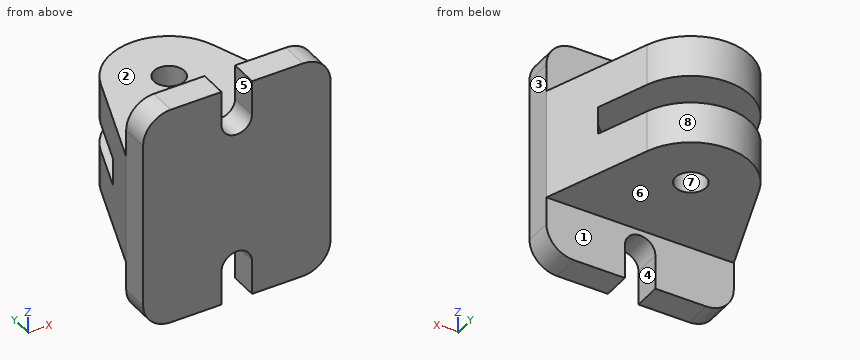
from build123d import *

# Parameters (mm, degrees)
SKETCH1_R           = 2.75
BOSS_EXTRUDE1_DEPTH = 10
SKETCH2_R           = 14.5
CUT_EXTRUDE1_DEPTH  = 2.5
BOSS_EXTRUDE2_DEPTH = 5
CUT_EXTRUDE5_DEPTH  = 41.387552571


with BuildPart() as part:
    # Sketch1 → Boss-Extrude1 (new, symmetric)
    with BuildSketch(Plane.XY):
        with BuildLine():
            Line((-10.101695673, 3.676716541), (-16.899464568, -15))
            Line((-16.899464568, -15), (16.899464568, -15))
            Line((16.899464568, -15), (10.101695673, 3.676716541))
            ThreePointArc((10.101695673, 3.676716541), (0, 10.75), (-10.101695673, 3.676716541))
        make_face()
        Circle(SKETCH1_R, mode=Mode.SUBTRACT)
    extrude(amount=BOSS_EXTRUDE1_DEPTH, both=True)

    # Sketch2 → Cut-Extrude1 (cut, symmetric)
    with BuildSketch(Plane.XY):
        Circle(SKETCH2_R)
    extrude(amount=CUT_EXTRUDE1_DEPTH, both=True, mode=Mode.SUBTRACT)

    # Sketch3 → Boss-Extrude2 (add)
    with BuildSketch(Plane.XZ.offset(15)):
        with BuildLine():
            Line((-16.899464568, 15), (-16.899464568, 10))
            Line((-16.899464568, 10), (16.899464568, 10))
            Line((16.899464568, 10), (16.899464568, 15))
            ThreePointArc((16.899464568, 15), (15.434998474, 18.535533906), (11.899464568, 20))
            Line((11.899464568, 20), (-11.899464568, 20))
            ThreePointArc((-11.899464568, 20), (-15.434998474, 18.535533906), (-16.899464568, 15))
        make_face()
        Polygon((16.899464568, 10), (-16.899464568, 10), (-16.899464568, -10), (16.899464568, -10), (16.899464568, 0), align=None)
        with BuildLine():
            Line((16.899464568, -10), (-16.899464568, -10))
            Line((-16.899464568, -10), (-16.899464568, -15))
            ThreePointArc((-16.899464568, -15), (-15.434998474, -18.535533906), (-11.899464568, -20))
            Line((-11.899464568, -20), (11.899464568, -20))
            ThreePointArc((11.899464568, -20), (15.434998474, -18.535533906), (16.899464568, -15))
            Line((16.899464568, -15), (16.899464568, -10))
        make_face()
    extrude(amount=BOSS_EXTRUDE2_DEPTH)

    # Sketch4 → Cut-Extrude5 (cut, through all)
    with BuildSketch(Plane.XZ.offset(20)):
        with BuildLine():
            Line((-2.75, 20), (-2.75, 13.75))
            ThreePointArc((-2.75, 13.75), (0, 11), (2.75, 13.75))
            Line((2.75, 13.75), (2.75, 20))
            Line((2.75, 20), (-2.75, 20))
        make_face()
        with BuildLine():
            Line((-2.75, -20), (-2.75, -13.75))
            ThreePointArc((-2.75, -13.75), (0, -11), (2.75, -13.75))
            Line((2.75, -13.75), (2.75, -20))
            Line((2.75, -20), (-2.75, -20))
        make_face()
    extrude(amount=-CUT_EXTRUDE5_DEPTH, mode=Mode.SUBTRACT)


solid = part.part
Verification items for the finished model (mm, model axes). Face numbers are marked on the shaded views. A direction names the side the tool comes from. Give positions to 0.01 mm unless a question says otherwise; leave off trailing zeros. Loops run counter-clockwise (first coordinate to the right, second up) from the corner with the lowest first, then second, coordinate; pieces in that order, holes last.
1. Cross-section at A-A on x = 0. Record the cut outline in (y, z), and give its area (3 significant figures).
Derived:
outline: (-20, -11) - (-15, -11) - (-15, -10) - (-2.75, -10) - (-2.75, -2.5) - (-14.5, -2.5) - (-14.5, 2.5) - (-2.75, 2.5) - (-2.75, 10) - (-15, 10) - (-15, 11) - (-20, 11) - close; (2.75, -10) - (10.75, -10) - (10.75, -2.5) - (2.75, -2.5) - close; (2.75, 2.5) - (10.75, 2.5) - (10.75, 10) - (2.75, 10) - close
area: 416 mm2
2. Cross-section at B-B on z = 9.5. Record the cut outline in (x, y), and give its area (3 significant figures).
Derived:
outline: (-16.9, -20) - (16.9, -20) - (16.9, -15) - (10.1, 3.68) arc R10.75 ccw to (-10.1, 3.68) - (-16.9, -15) - close; hole circle Ø5.5 at (0, 0)
area: 754 mm2
3. Go/stop test with flat-tipped pins: P1, Ø3, axis at x = -0.5, z = 14, coming from the +Y side; P2, Ø1.5, axis at y = -11, z = -5.5, coming from the +X side; P3, Ø10, axis at y = 0, z = -4.5, coming from the +X side; P4, Ø4, axis at x = 8.5, z = -5.5, coming from the +Y side. Record where each tip stops, or that it passes through.
Derived:
P1: passes through
P2: stops at x = 15.72
P3: stops at x = 13.26
P4: stops at y = 8.56
4. Cross-section at D-D on z = -16. Record the cut outline in (x, y).
Derived:
outline: (-16.8, -20) - (-2.75, -20) - (-2.75, -15) - (-16.8, -15) - close; (2.75, -20) - (16.8, -20) - (16.8, -15) - (2.75, -15) - close
5. Cross-section at C-C on y = 4.5. Record the cut outline in (x, z), and give its area (3 significant figures).
Derived:
outline: (-9.76, -10) - (9.76, -10) - (9.76, -2.5) - (-9.76, -2.5) - close; (-9.76, 2.5) - (9.76, 2.5) - (9.76, 10) - (-9.76, 10) - close
area: 293 mm2
6. Release check for a two-part mould opening along X. For the marked faces 6, 7 and 8 record: +X half, -X half, draft (parallel to the pull), parting line (faces both ways), or undercut.
Derived:
face 6: draft
face 7: undercut
face 8: parting line
7. Tool access check on the marked faces 1, 2, 3, 4 and 5. Record the directions out of +Z, -Z, +X, -X, +Y, -Y that give a thin tool (end or side, any length) a straight path to the whole face; none if there is none.
Derived:
face 1: -Z, +X, -X, +Y
face 2: +Z, +X, -X, +Y
face 3: +Z, -Z, +X, +Y, -Y
face 4: -Z, +Y, -Y
face 5: +Z, +Y, -Y
8. Material ranges on probe 1 along Z at (x, y) = (-7, -12); probe 2 along Y at (x, z) = (3.5, 13); probe 3 along Z at (x, y) = (14, -13), recorded low to high.
Derived:
probe 1: z = -10 to -2.5, 2.5 to 10
probe 2: y = -20 to -15
probe 3: z = -10 to 10
